from build123d import *

# Parameters (mm, degrees)
SKETCH_1_W          = 250
SKETCH_1_H          = 250
EXTRUDE_1_DEPTH     = 10
SKETCH_2_R          = 5
EXTRUDE_2_DEPTH     = 10
SKETCH_3_R          = 5
EXTRUDE_3_DEPTH     = 30
SKETCH_4_W          = 14.8
SKETCH_4_H          = 165
EXTRUDE_4_DEPTH     = 20
SKETCH_5_W          = 100
SKETCH_5_H          = 65
EXTRUDE_5_DEPTH     = 20
SKETCH_6_W          = 100
SKETCH_6_H          = 250
EXTRUDE_6_DEPTH     = 10
SKETCH_7_W          = 70.2
SKETCH_7_H          = 165
EXTRUDE_7_DEPTH     = 10
SKETCH_8_W          = 30
SKETCH_8_H          = 120
EXTRUDE_8_DEPTH     = 20
SKETCH_9_W          = 30
SKETCH_9_H          = 20
CUT_EXTRUDE_1_DEPTH = 10


with BuildPart() as part:
    # 草图1 → 凸台-拉伸1 (new body)
    with BuildSketch(Plane.XY):
        Rectangle(SKETCH_1_W, SKETCH_1_H)
    extrude(amount=-EXTRUDE_1_DEPTH)

    # 草图2 → 凸台-拉伸2 (add)
    with BuildSketch(Plane.XY):
        with Locations((-68.35, 40)):
            Circle(SKETCH_2_R)
    extrude_2 = extrude(amount=EXTRUDE_2_DEPTH)

    # 镜向1: 凸台-拉伸2 across plane
    add(extrude_2.mirror(Plane.ZX))

    # 草图3 → 凸台-拉伸3 (add)
    with BuildSketch(Plane.XY):
        with Locations((0, 40)):
            Circle(SKETCH_3_R)
    extrude(amount=EXTRUDE_3_DEPTH)

    # 草图4 → 凸台-拉伸4 (add)
    with BuildSketch(Plane.XY):
        with Locations((27.4, 42.5)):
            Rectangle(SKETCH_4_W, SKETCH_4_H)
    extrude(amount=EXTRUDE_4_DEPTH)

    # 草图5 → 凸台-拉伸5 (add)
    with BuildSketch(Plane.XY):
        with Locations((75, -92.5)):
            Rectangle(SKETCH_5_W, SKETCH_5_H)
    extrude(amount=EXTRUDE_5_DEPTH)

    # 草图6 → 凸台-拉伸6 (add)
    with BuildSketch(Plane.XY):
        with Locations((75, 0)):
            Rectangle(SKETCH_6_W, SKETCH_6_H)
    extrude(amount=EXTRUDE_6_DEPTH)

    # 草图7 → 凸台-拉伸7 (add)
    with BuildSketch(Plane.XY.offset(10)):
        with Locations((89.9, 42.5)):
            Rectangle(SKETCH_7_W, SKETCH_7_H)
    extrude(amount=EXTRUDE_7_DEPTH)

    # 草图8 → 凸台-拉伸8 (add)
    with BuildSketch(Plane.XY):
        with Locations((10, -65)):
            Rectangle(SKETCH_8_W, SKETCH_8_H)
    extrude(amount=EXTRUDE_8_DEPTH)

    # 草图9 → 切除-拉伸1 (cut)
    with BuildSketch(Plane.XY.offset(20)):
        with Locations((10, -50)):
            Rectangle(SKETCH_9_W, SKETCH_9_H)
    extrude(amount=-CUT_EXTRUDE_1_DEPTH, mode=Mode.SUBTRACT)


solid = part.part
Geometry check sheet. Reference: the model listing, model coordinates, mm. A direction names the side the tool comes from. Give positions to 0.01 mm unless a question says otherwise; leave off trailing zeros. Order: outer loops, then holes, each group sorted by start corner. A loop starts at its lowest first (then second) coordinate and runs counter-clockwise, first axis right, second up.
1) Cross-section at C-C (x = -68.35). Record the boundary of the cut face in (y, z), then the cut area to 3 significant figures.
Results are:
outline: (-125, -10) - (125, -10) - (125, 0) - (45, 0) - (45, 10) - (35, 10) - (35, 0) - (-35, 0) - (-35, 10) - (-45, 10) - (-45, 0) - (-125, 0) - close
area: 2,700 mm2
2) Tool access check on faces 5 (the cylindrical face through (-73.345, -40.22, 4.93)), 6 (the flat face through (54.8, 41, 15)), 7 (the flat face through (0, 40, 30)), 8 (the flat face through (-68, -40, 10)). Record the directions out of +Z, -Z, +X, -X, +Y, -Y that give a thin tool (end or side, any length) a straight path to the whole face; none if there is none.
Results are:
face 5: +Z
face 6: +Z, +Y
face 7: +Z, +X, -X, +Y, -Y
face 8: +Z, -X, +Y, -Y
3) Gauge pin test, flat ends, axial feed: pin 1 (8 mm diameter, centred on y = 4.5, z = 14, fed in from -X); pin 2 (6 mm diameter, centred on x = 38.5, y = -19, fed in from +Z); pin 3 (10 mm diameter, centred on y = -64, z = 11.5, fed in from -X). Record the tip position at first contact, or that the pin passes through.
Results are:
pin 1: stops at x = 20
pin 2: stops at z = 10
pin 3: stops at x = -5
4) Cross-section at D-D (x = 0). Record the boundary of the cut face in (y, z).
Results are:
outline: (-125, -10) - (125, -10) - (125, 0) - (45, 0) - (45, 30) - (35, 30) - (35, 0) - (-5, 0) - (-5, 20) - (-40, 20) - (-40, 10) - (-60, 10) - (-60, 20) - (-125, 20) - close
5) Material ranges on probe 1 along Y at (x, z) = (10, 14.5); probe 2 along X at (y, z) = (50, 17); probe 3 along X at (y, z) = (38, 10.5), recorded low to high.
Results are:
probe 1: y = -125 to -60, -40 to -5
probe 2: x = 20 to 34.8, 54.8 to 125
probe 3: x = -4.58 to 4.58, 20 to 34.8, 54.8 to 125
6) Draft check along X on faces 1 (the flat face through (34.8, 41, 15)), 2 (the flat face through (125, -2, 5)), 3 (the flat face through (59, -60, 15)), 4 (the flat face through (-125, -2, -5)). Enter one of: released by +X, released by -X, zero draft, split by the parting line, or undercut.
Results are:
face 1: undercut
face 2: released by +X
face 3: zero draft
face 4: released by -X
7) Cross-section at B-B (y = 40). Record the boundary of the cut face in (x, z).
Results are:
outline: (-125, -10) - (125, -10) - (125, 20) - (54.8, 20) - (54.8, 10) - (34.8, 10) - (34.8, 20) - (20, 20) - (20, 0) - (5, 0) - (5, 30) - (-5, 30) - (-5, 0) - (-63.35, 0) - (-63.35, 10) - (-73.35, 10) - (-73.35, 0) - (-125, 0) - close
8) Cross-section at A-A (z = 13). Record the boundary of the cut face in (x, y), then the cut area to 3 significant figures.
Results are:
outline: (-5, -125) - (125, -125) - (125, -60) - (-5, -60) - close; (-5, -40) - (34.8, -40) - (34.8, 125) - (20, 125) - (20, -5) - (-5, -5) - close; circle Ø10 at (0, 40); (54.8, -40) - (125, -40) - (125, 125) - (54.8, 125) - close
area: 23,400 mm2
